Source: three-view drawing plus pictorial views. Frame: mm from the lowest corner of the part. Coordinates: 2 decimals unless noted, no trailing zeros. Write each loop counter-clockwise with the first axis right and the second up, starting at its lowest first coordinate (ties: lowest second). Pieces come first, ordered by that corner, then holes. Notation, with made-up numbers: (42, -7.5) -> (93, -7.5) arc R18 cw to (93, 5.5) -> close; hole circle Ø3 at (43, 72). An arc over 180 degrees is marked (long way). Write item = value, one per line.
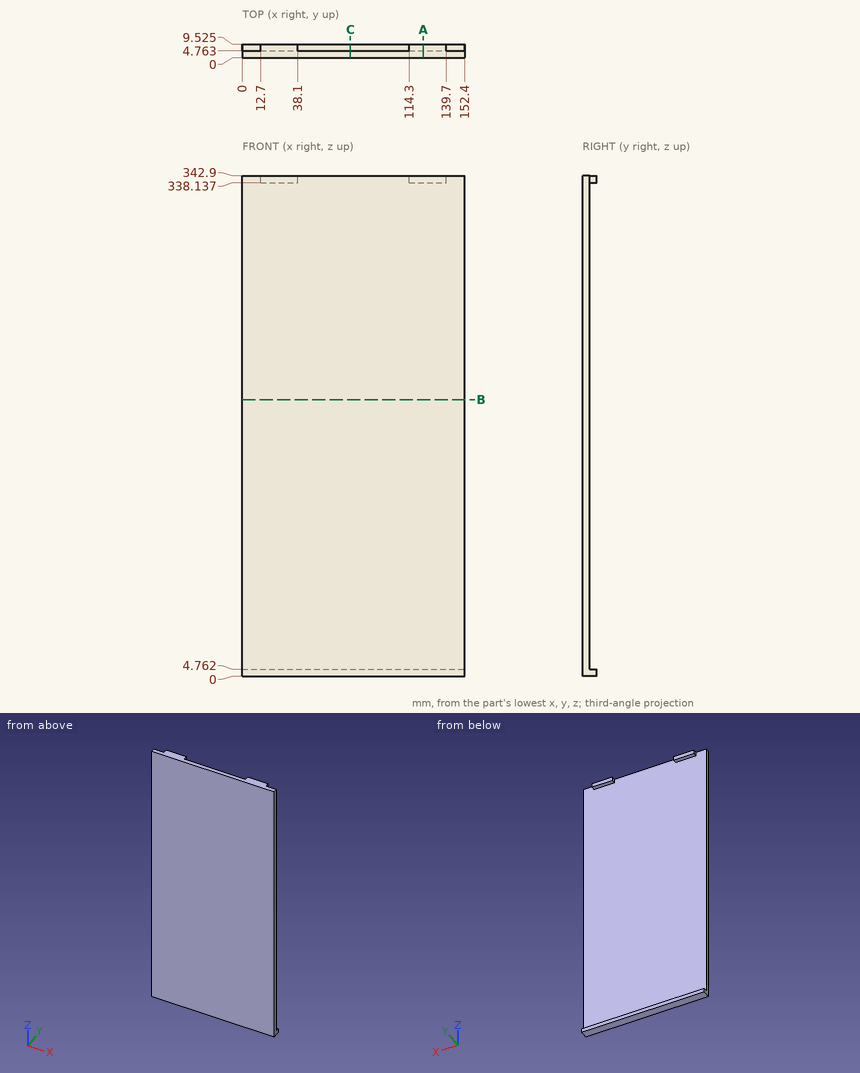
1) Cut plane A-A, the plane x = 124. Output: boundary loops of the cut face in (y, z) (1 decimal), and give its area (3 significant figures).
Answer block:
outline = (0, 0) -> (9.5, 0) -> (9.5, 4.8) -> (4.8, 4.8) -> (4.8, 338.1) -> (9.5, 338.1) -> (9.5, 342.9) -> (0, 342.9) -> close
area = 1,680 mm2
2) Material intervals for probe 1 along Z at (x, y) = (102, 7.75); probe 2 along Z at (x, y) = (16, 9.25), sorted ascending. Write a range as [from, to].
Answer block:
probe_1 = [0, 4.76]
probe_2 = [0, 4.76], [338.14, 342.9]
3) Cut plane B-B, the plane z = 189.5. Output: boundary loops of the cut face in (x, y).
Answer block:
outline = (0, 0) -> (152.4, 0) -> (152.4, 4.76) -> (0, 4.76) -> close
4) Cut plane C-C, the plane x = 74. Output: boundary loops of the cut face in (y, z) (1 decimal), and give its area (3 significant figures).
Answer block:
outline = (0, 0) -> (9.5, 0) -> (9.5, 4.8) -> (4.8, 4.8) -> (4.8, 342.9) -> (0, 342.9) -> close
area = 1,660 mm2
5) First-contact query: pin 1 Ø12 at (x, z) = (57, 124) entering from +Y; pin 2 Ø1.4 at (y, z) = (7, 341.5) entering from +X; pin 3 Ø2.5 at (y, z) = (6.5, 341.5) entering from -X. Flat tips, straight axial feed; report the tip coordinate or a pass-through.
Answer block:
pin_1 = 4.76
pin_2 = 139.7
pin_3 = 12.7
